Autodesk Fusion 360 part; units mm, degrees
sketch "Sketch3" plane through (0, 0, 0) normal (0, 1, 0) x (1, 0, 0)
  line L0 (0, 0) -> (-77.216, 0)
  line L1 (-77.216, 0) -> (-77.216, -38.1)
  line L2 (-77.216, -38.1) -> (-39.116, -38.1)
  line L3 (-39.116, -38.1) -> (-39.116, -95.25)
  line L4 (-39.116, -95.25) -> (-77.216, -95.25)
  line L5 (-77.216, -95.25) -> (-77.216, -120.65)
  line L6 (-77.216, -120.65) -> (-30.4714, -120.65)
  line L7 (-0.0056, -121.5825) -> (0, 0)
  line L8 (-30.4714, -120.65) -> (-30.4714, -178.7325)
  line L9 (-30.4714, -178.7325) -> (-0.0056, -178.7325)
  line L10 (-0.0056, -178.7325) -> (-0.0056, -121.5825)
  dimension "d9" = 77.216
  dimension "d10" = 38.1
  dimension "d11" = 38.1
  dimension "d12" = 57.15
  dimension "d13" = 38.1
  dimension "d14" = 25.4
  dimension "d15" = 77.216
  dimension "d17" = 57.15
extrude "Extrude2" add sketch "Sketch3" along normal blind 95.25
Work out the finished part from the listing and answer in its coordinate system (mm). A direction names the side the tool comes from. Round coordinates to 2 decimals unless told otherwise and drop trailing zeros. Loops run counter-clockwise (first coordinate to the right, second up) from the corner with the lowest first, then second, coordinate; pieces in that order, holes last.
(1) Each of these flat-tipped pins is pushed along its axis until it touches: P1, Ø19, axis at x = -57.5, y = 26, coming from the +Z side; P2, Ø4, axis at y = 20, z = 47, coming from the -X side. Where does it stop, or does it pass through?
Computed values:
P1: stops at z = 120.65
P2: stops at x = -39.12
(2) The part is cut by section C-C, the plane z = 145. Give the vertices of the cut face in (x, y), and give its area (3 significant figures).
Computed values:
outline: (-30.47, 0) - (-0.01, 0) - (-0.01, 95.25) - (-30.47, 95.25) - close
area: 2,900 mm2
(3) Find the intervals of material crossed by L1, parallel to Z at x = -52.5, y = 34; L2, parallel to X at y = 44, z = 144; L3, parallel to X at y = 40.5, z = 27.5, in increasing order.
Computed values:
L1: z = 0 to 38.1, 95.25 to 120.65
L2: x = -30.47 to -0.01
L3: x = -77.22 to 0
(4) The part is cut by section D-D, the plane z = 83. Give the vertices of the cut face in (x, y), and give its area (3 significant figures).
Computed values:
outline: (-39.12, 0) - (0, 0) - (0, 95.25) - (-39.12, 95.25) - close
area: 3,730 mm2
(5) For faces 4 (the flat face through (-30.471, 47, 149)), 5 (the flat face through (-77.216, 47, 19)), 6 (the flat face through (-58, 47, 95.25)), determine the directions among +Z, -Z, +X, -X, +Y, -Y from which every point of the face is accessible in a straight line to the end or side of a thin tool.
Computed values:
face 4: +Z, -X, +Y, -Y
face 5: +Z, -Z, -X, +Y, -Y
face 6: -X, +Y, -Y
(6) The part is cut by section A-A, the plane x = -60. Give the vertices of the cut face in (y, z), and give its area (3 significant figures).
Computed values:
outline: (0, 0) - (95.25, 0) - (95.25, 38.1) - (0, 38.1) - close; (0, 95.25) - (95.25, 95.25) - (95.25, 120.65) - (0, 120.65) - close
area: 6,050 mm2
(7) The mould has two halves that part along Z. Classify faces 1 (the flat face through (-31, 0, 68)), 2 (the flat face through (-54, 47, 120.65)), 3 (the flat face through (-39.116, 47, 66)): pulls with the +Z half, pulls with the -Z half, needs draft (parallel to the pull), parting line crosses it, or undercut.
Computed values:
face 1: needs draft
face 2: pulls with the +Z half
face 3: undercut
(8) The part is cut by section B-B, the plane y = 50.5. Give the vertices of the cut face in (x, z).
Computed values:
outline: (-77.22, 0) - (0, 0) - (-0.01, 121.58) - (-0.01, 178.73) - (-30.47, 178.73) - (-30.47, 120.65) - (-77.22, 120.65) - (-77.22, 95.25) - (-39.12, 95.25) - (-39.12, 38.1) - (-77.22, 38.1) - close
